Autodesk Inventor part; units mm, degrees
ref_plane "YZ Plane" through (0, 0, 0) normal (1, 0, 0) x (0, 1, 0)
ref_plane "XZ Plane" through (0, 0, 0) normal (0, 1, 0) x (-1, 0, 0)
ref_plane "XY Plane" through (0, 0, 0) normal (0, 0, 1) x (1, 0, 0)
sketch "Sketch1" plane through (0, 0, 0) normal (0, 0, 1) x (1, 0, 0)
  line L0 (-12.7, -12.7) -> (12.7, -12.7)
  line L1 (12.7, -12.7) -> (12.7, 12.7)
  line L2 (12.7, 12.7) -> (-12.7, 12.7)
  line L3 (-12.7, 12.7) -> (-12.7, -12.7)
  line L4 (-12.7, -12.7) -> (12.7, 12.7) construction
  line L5 (12.7, -12.7) -> (-12.7, 12.7) construction
  line L6 (-11.1125, 11.1125) -> (11.1125, 11.1125)
  line L7 (11.1125, 11.1125) -> (11.1125, -11.1125)
  line L8 (11.1125, -11.1125) -> (-11.1125, -11.1125)
  line L9 (-11.1125, -11.1125) -> (-11.1125, 11.1125)
  point P0 (0, 0)
  dimension "width" = 25.4
  dimension "height" = 25.4
  dimension "thickness" = 1.5875
extrude "Extrusion1" add sketch "Sketch1" along normal mid plane 304.8
sketch "Sketch2" plane through (12.7, -12.7, 152.4) normal (1, 0, 0) x (0, 0, -1)
  line L0 (304.8, 25.4) -> (304.8, 0) construction
  line L1 (304.8, 0) -> (0, 0) construction
  line L2 (0, 0) -> (0, 25.4) construction
  line L3 (0, 25.4) -> (304.8, 25.4) construction
  point P0 (152.4, 12.7)
  point P1 (292.1, 12.7)
  point P2 (304.8, 12.7)
  point P3 (266.7, 12.7)
  dimension "d5" = 12.7
  dimension "d6" = 25.4
hole "Hole1" at (12.7, 0, -139.7) at (12.7, 0, -114.3) direction (-1, 0, 0) diameter 5.1054 end through all
sketch "Sketch3" plane through (-12.7, 12.7, 152.4) normal (0, 1, 0) x (1, 0, 0)
  line L0 (25.4, 0) -> (0, 0) construction
  point P0 (12.7, 152.4)
  point P1 (14.2875, 7.9502)
  point P2 (14.2875, 42.8752)
  point P3 (12.7, 0)
  point P4 (12.7, 0)
  dimension "d14" = 34.925
  dimension "d32" = 7.9502
  dimension "d33" = 1.5875
hole "Hole2" at (1.5875, 12.7, 144.4498) at (1.5875, 12.7, 109.5248) direction (0, -1, 0) diameter 5.1054 end through all
sketch "Sketch4" plane through (-12.7, -12.7, 152.4) normal (-1, 0, 0) x (0, 0, 1)
  line L0 (-139.7, 12.7) -> (-25.4, 12.7) construction
  line L1 (0, 25.4) -> (0, 0) construction
  point P0 (-152.4, 12.7)
  point P1 (-82.55, 12.7)
  point P2 (-82.55, 12.7)
  dimension "d23" = 25.4
  dimension "d24" = 114.3
hole "Hole3" at (-12.7, 0, 127) at (-12.7, 0, 69.85) at (-12.7, 0, 12.7) direction (1, 0, 0) diameter 5.1054 end through all
sketch "Sketch5" plane through (12.7, -12.7, 152.4) normal (1, 0, 0) x (0, 0, -1)
  line L0 (304.8, 25.4) -> (0, 25.4) construction
  line L1 (304.8, 25.4) -> (304.8, 0) construction
  point P0 (152.4, 12.7)
  point P1 (196.85, 12.7)
  point P2 (234.95, 12.7)
  dimension "d34" = 38.1
  dimension "d35" = 12.7
  dimension "d36" = 69.85
hole "Hole4" at (12.7, 0, -44.45) at (12.7, 0, -82.55) direction (-1, 0, 0) diameter 4.4958 end through all
properties part number "CL4-002" material "Aluminum 6061"
Geometry check sheet. Reference: the model listing, model coordinates, mm. A direction names the side the tool comes from. Give positions to 0.01 mm unless a question says otherwise; leave off trailing zeros. Loops run counter-clockwise (first coordinate to the right, second up) from the corner with the lowest first, then second, coordinate; pieces in that order, holes last.
(1) Set-up check for faces 4 (the cylindrical face through (-11.92, -0.11, -111.75)), 5 (the flat face through (-11.112, 0, -2)): record each of +Z, -Z, +X, -X, +Y, -Y from which the full face is reachable in a straight line by a thin tool's end or side.
From the geometry:
face 4: +X, -X
face 5: +Z, -Z
(2) Release check for a two-part mould opening along Z. For faces 1 (the flat face through (-11.3, 0.1, 152.4)), 2 (the cylindrical face through (11.9, -0.11, -111.75)), 3 (the flat face through (-12.7, 0, -2)) record: released by +Z, released by -Z, zero draft, split by the parting line, or undercut.
From the geometry:
face 1: released by +Z
face 2: undercut
face 3: zero draft
(3) Depth check by flat-ended pin: pin 1 Ø3 at (x, y) = (-8, 3.5) entering from -Z; pin 2 Ø8 at (x, z) = (1.59, 144.45) entering from +Y. Enter the tip coordinate at first touch or a pass-through.
From the geometry:
pin 1: passes through
pin 2: stops at y = 12.7
(4) Section check A-A on z = -139.7. Record the cut outline in (x, y).
From the geometry:
outline: (-12.7, -12.7) - (12.7, -12.7) - (12.7, -2.55) - (11.11, -2.55) - (11.11, -11.11) - (-11.11, -11.11) - (-11.11, -2.55) - (-12.7, -2.55) - close; (-12.7, 2.55) - (-11.11, 2.55) - (-11.11, 11.11) - (11.11, 11.11) - (11.11, 2.55) - (12.7, 2.55) - (12.7, 12.7) - (-12.7, 12.7) - close
(5) Section check B-B on y = -6. Record the cut outline in (x, z), then the cut area to 3 significant figures.
From the geometry:
outline: (-12.7, -152.4) - (-11.11, -152.4) - (-11.11, 152.4) - (-12.7, 152.4) - close; (11.11, -152.4) - (12.7, -152.4) - (12.7, 152.4) - (11.11, 152.4) - close
area: 968 mm2
(6) Section check D-D on z = 102.5. Record the cut outline in (x, y).
From the geometry:
outline: (-12.7, -12.7) - (12.7, -12.7) - (12.7, 12.7) - (-12.7, 12.7) - close; hole (-11.11, -11.11) - (11.11, -11.11) - (11.11, 11.11) - (-11.11, 11.11) - close
(7) Thickness scan on L1, parallel to Y at x = -11.85, z = -139.7; L2, parallel to X at y = 9.5, z = -132. Record the ranges inside material, lowest first.
From the geometry:
L1: y = -12.7 to -2.55, 2.55 to 12.7
L2: x = -12.7 to -11.11, 11.11 to 12.7
